```python
from build123d import *

# Parameters (mm, degrees)
SKETCH12_W         = 0.866666667
SKETCH12_H         = 0.866666667
CHAMFER3_SIZE      = 0.26
CHAMFER1_SIZE      = 0.75
CHAMFER2_SIZE      = 0.4225
CUT_EXTRUDE2_DEPTH = 3


with BuildPart() as part:
    # Sketch1 → Revolve1 (revolve)
    with BuildSketch(Plane(origin=(0, 0, 0), x_dir=(0, 0, -1), z_dir=(1, 0, 0))):
        Polygon((0, 6.5), (6, 6.5), (6, 4), (51, 4), (51, 3), (62, 3), (62, 0), (0, 0), align=None)
    revolve(axis=Axis((0, 0, -62), (0, 0, 1)))

    # Sketch12 → Cut-Revolve2 (revolve, cut)
    with BuildSketch(Plane(origin=(0, 0, 0), x_dir=(0, 0, -1), z_dir=(1, 0, 0))):
        with Locations((6.433333334, 3.566666667)):
            Rectangle(SKETCH12_W, SKETCH12_H)
    revolve(axis=Axis((0, 0, -62), (0, 0, 1)), mode=Mode.SUBTRACT)

    # Chamfer3
    chamfer3_edges = [part.edges().sort_by_distance(p)[0] for p in [
        (0, -3.133333333, -6.866666667),
        (0, -4, -6.866666667),
    ]]
    chamfer(chamfer3_edges, length=CHAMFER3_SIZE)

    # Sketch5 → Cut-Revolve1 (revolve, cut)
    with BuildSketch(Plane(origin=(0, 0, 0), x_dir=(0, 0, -1), z_dir=(1, 0, 0))):
        with BuildLine():
            Line((51, 4), (55.4, 4))
            Line((55.4, 4), (53.6, 2.2))
            Line((53.6, 2.2), (51.8, 2.2))
            ThreePointArc((51.8, 2.2), (51.234314575, 2.434314575), (51, 3))
            Line((51, 3), (51, 4))
        make_face()
    revolve(axis=Axis((0, 0, -62), (0, 0, 1)), mode=Mode.SUBTRACT)

    # Chamfer1
    chamfer1_edges = [part.edges().sort_by_distance(p)[0] for p in [
        (0, -3, -62),
    ]]
    chamfer(chamfer1_edges, length=CHAMFER1_SIZE)

    # Chamfer2
    chamfer2_edges = [part.edges().sort_by_distance(p)[0] for p in [
        (0, -4, -51),
        (0, -6.5, 0),
    ]]
    chamfer(chamfer2_edges, length=CHAMFER2_SIZE)

    # Sketch8 → Cut-Extrude2 (cut)
    with BuildSketch(Plane.XY):
        Polygon((2, 1.154700538), (0, 2.309401077), (-2, 1.154700538), (-2, -1.154700538), (0, -2.309401077), (2, -1.154700538), align=None)
    extrude(amount=-CUT_EXTRUDE2_DEPTH, mode=Mode.SUBTRACT)

    # Cut-Extrude4 cone 1 section (through the dimple's axis) → Cut-Extrude4 (revolve, cut)
    with BuildSketch(Plane(origin=(0, 0, 0), x_dir=(0, -1, 0), z_dir=(1, 0, 0))):
        Polygon((0, 0), (2.309401077, 0), (0, 2.309401077), align=None)
    revolve(axis=Axis((0, 0, 0), (0, 0, -1)), mode=Mode.SUBTRACT)


solid = part.part
```
The model under review builds one solid part; all positions refer to its coordinate system, in mm. A direction names the side the tool comes from. Round coordinates to 2 decimals unless told otherwise and drop trailing zeros. Order: outer loops, then holes, each group sorted by start corner. A loop starts at its lowest first (then second) coordinate and runs counter-clockwise, first axis right, second up. Notation, with made-up numbers: (-32.75, 45.5) - (-5.75, 45.5) arc R27 ccw to (-5.75, 66.5) - close; hole circle Ø10 at (34.5, 21.25). An arc over 180 degrees is marked (long way). Answer in a Markdown table with one row per item.
(1) Mouldability with a two-part tool opening along Y and no side actions: class faces 4 (the face through (-1.06, -1.87, -0.16)), 5 (the face through (0, 0, -62)), 6 (the face through (2.78, 1.446, -6.308)) as released by +Y, released by -Y, zero draft, split by the parting line, or undercut.
Result set:
| item | result |
|---|---|
| face 4 | undercut |
| face 5 | zero draft |
| face 6 | split by the parting line |
(2) For line 1 (Z direction, x = 2, y = -2.75); line 2 (Z direction, x = 0, y = -1.75); line 3 (Y direction, x = -2.5, z = -38.5), list the stretches that pass through material, from the lowest coordinate up. Write a range as from..to.
Result set:
| item | result |
|---|---|
| line 1 | z = -51..-6.87, -6..0 |
| line 2 | z = -62..-3 |
| line 3 | y = -3.12..3.12 |
(3) Take a section at A-A on z = -53. Write out the cut boundary in (x, y).
Result set:
| item | result |
|---|---|
| outline | circle Ø4.4 at (0, 0) |
(4) Machinability: for faces 1 (the face through (0, -3, 0)), 2 (the face through (1.06, 1.87, -0.16)), 3 (the face through (-0.66, 2.1, -52.69)), which of the approach directions +Z, -Z, +X, -X, +Y, -Y give a long, thin tool a straight path to every point of the face, cutting with its end or side? Answer none if there is none.
Result set:
| item | result |
|---|---|
| face 1 | +Z, +X, -X, +Y, -Y |
| face 2 | +Z |
| face 3 | none |
(5) Clearance check with flat-ended pins moving along their axes: P1, Ø5, axis at x = 1, z = -11.5, coming from the +Y side; P2, Ø1, axis at y = 5, z = -48.5, coming from the -X side; P3, Ø1.5, axis at y = -4, z = -24, coming from the +X side; P4, Ø4, axis at y = -1, z = -41, coming from the -X side. State where each tip first meets the part, or that it passes through.
Result set:
| item | result |
|---|---|
| P1 | stops at y = 4 |
| P2 | passes through |
| P3 | stops at x = 2.33 |
| P4 | stops at x = -4 |
